Source: CAD feature listing. Evaluate the final solid. Frame: model axes, mm. Give positions to 0.01 mm unless a question says otherwise; leave off trailing zeros. Order: outer loops, then holes, each group sorted by start corner. A loop starts at its lowest first (then second) coordinate and runs counter-clockwise, first axis right, second up. Notation, with made-up numbers: M 28.5,18.25 L 80.5,18.25 A30 cw 80.5,40.25 Z; hole C 51.5,55 d5. An arc over 180 degrees is marked long. Return JSON: item names as keys, results as strings.
from build123d import *

# Parameters (mm, degrees)
SKETCH2_W           = 20
SKETCH2_H           = 20
BOSS_EXTRUDE1_DEPTH = 20
SKETCH3_R           = 2
CUT_EXTRUDE2_DEPTH  = 1.5
SKETCH4_R           = 2
CUT_EXTRUDE4_DEPTH  = 1.5
SKETCH5_R           = 2
CUT_EXTRUDE5_DEPTH  = 1.5
SKETCH6_R           = 2
CUT_EXTRUDE6_DEPTH  = 1.5
SKETCH7_R           = 2
CUT_EXTRUDE7_DEPTH  = 1.5
SKETCH8_R           = 2
CUT_EXTRUDE8_DEPTH  = 1.5
SKETCH9_R           = 2
CUT_EXTRUDE9_DEPTH  = 1.5


with BuildPart() as part:
    # Sketch2 → Boss-Extrude1 (new body)
    with BuildSketch(Plane.XY):
        with Locations((0, 10)):
            Rectangle(SKETCH2_W, SKETCH2_H)
    extrude(amount=BOSS_EXTRUDE1_DEPTH)

    # Sketch3 → Cut-Extrude2 (cut)
    with BuildSketch(Plane(origin=(0, 0, 0), x_dir=(-1, 0, 0), z_dir=(0, 0, -1))):
        with Locations((0, 11.387488096)):
            Circle(SKETCH3_R)
    extrude(amount=-CUT_EXTRUDE2_DEPTH, mode=Mode.SUBTRACT)

    # Sketch4 → Cut-Extrude4 (cut)
    with BuildSketch(Plane.XY.offset(20)):
        with Locations((-6.679680773, 3.199433654)):
            Circle(SKETCH4_R)
        with Locations((-6.679680773, 9.585684456)):
            Circle(SKETCH4_R)
        with Locations((-6.679680773, 15.895974219)):
            Circle(SKETCH4_R)
        with Locations(Location((5.94831499, 16.092405647, 0), (0, 0, 180))):
            Circle(SKETCH4_R)
        with Locations(Location((6.144583567, 9.785168888, 0), (0, 0, 180))):
            Circle(SKETCH4_R)
        with Locations(Location((6.343214755, 3.402007841, 0), (0, 0, 180))):
            Circle(SKETCH4_R)
    extrude(amount=-CUT_EXTRUDE4_DEPTH, mode=Mode.SUBTRACT)

    # Sketch5 → Cut-Extrude5 (cut)
    with BuildSketch(Plane.XZ):
        with Locations(Location((-7.031123571, 4.41764723, 0), (0, 0, 270))):
            Circle(SKETCH5_R)
        with Locations(Location((-7.031123571, 13.242962798, 0), (0, 0, 270))):
            Circle(SKETCH5_R)
        with Locations(Location((7.031123571, 13.242962798, 0), (0, 0, 90))):
            Circle(SKETCH5_R)
        with Locations(Location((7.031123571, 4.41764723, 0), (0, 0, 90))):
            Circle(SKETCH5_R)
    extrude(amount=-CUT_EXTRUDE5_DEPTH, mode=Mode.SUBTRACT)

    # Sketch6 → Cut-Extrude6 (cut)
    with BuildSketch(Plane(origin=(0, 20, 0), x_dir=(1, 0, 0), z_dir=(0, 1, 0))):
        with Locations(Location((-6.836211915, -14.945689643, 0), (0, 0, 270))):
            Circle(SKETCH6_R)
        with Locations(Location((3.056286481, -5.000631722, 0), (0, 0, 270))):
            Circle(SKETCH6_R)
    extrude(amount=-CUT_EXTRUDE6_DEPTH, mode=Mode.SUBTRACT)

    # Sketch7 → Cut-Extrude7 (cut)
    with BuildSketch(Plane.ZY.offset(10)):
        with Locations((15.664719218, 3.42791907)):
            Circle(SKETCH7_R)
        with Locations((6.506483369, 3.42791907)):
            Circle(SKETCH7_R)
        with Locations(Location((6.506483369, 15.851101107, 0), (0, 0, 180))):
            Circle(SKETCH7_R)
        with Locations(Location((15.664719218, 15.851101107, 0), (0, 0, 180))):
            Circle(SKETCH7_R)
    extrude(amount=-CUT_EXTRUDE7_DEPTH, mode=Mode.SUBTRACT)

    # Sketch8 → Cut-Extrude8 (cut)
    with BuildSketch(Plane.ZY.offset(10)):
        with Locations((10.73729624, 9.476774356)):
            Circle(SKETCH8_R)
    extrude(amount=-CUT_EXTRUDE8_DEPTH, mode=Mode.SUBTRACT)

    # Sketch9 → Cut-Extrude9 (cut)
    with BuildSketch(Plane(origin=(10, 0, 0), x_dir=(0, 0, -1), z_dir=(1, 0, 0))):
        with Locations((-16.749886235, 16.691371863)):
            Circle(SKETCH9_R)
        with Locations((-10.039394763, 9.986036972)):
            Circle(SKETCH9_R)
        with Locations((-4.265304833, 3.925944784)):
            Circle(SKETCH9_R)
    extrude(amount=-CUT_EXTRUDE9_DEPTH, mode=Mode.SUBTRACT)


solid = part.part
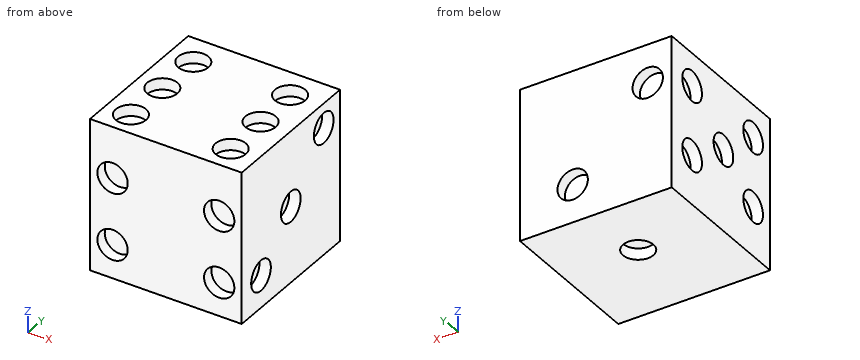
1. Ray query, probe 1 along Z at (x, y) = (5.75, 10.25); probe 2 along Y at (x, z) = (7, 14.25); probe 3 along X at (y, z) = (5.5, 3.5). Return the intervals inside material, ascending.
Evaluation:
{"probe 1": "z = 0 to 18.5", "probe 2": "y = 1.5 to 20", "probe 3": "x = -10 to 8.5"}
2. Section query A-A (x = 0). Return loops of the section in (y, z).
Evaluation:
{"outline": "M 0,0 L 9.39,0 L 9.39,1.5 L 13.39,1.5 L 13.39,0 L 20,0 L 20,20 L 0,20 Z"}
3. Section query B-B (y = 9). Return loops of the section in (x, z).
Evaluation:
{"outline": "M -10,0 L 10,0 L 10,8.3 L 8.5,8.3 L 8.5,11.78 L 10,11.78 L 10,20 L 7.98,20 L 7.98,18.5 L 4.31,18.5 L 4.31,20 L -4.77,20 L -4.77,18.5 L -8.59,18.5 L -8.59,20 L -10,20 L -10,12.68 L -8.5,12.68 L -8.5,8.79 L -10,8.79 Z"}
4. Section query C-C (z = 16). Return loops of the section in (x, y), then the cut area to 3 significant figures.
Evaluation:
{"outline": "M -10,0 L 10,0 L 10,14.84 L 8.5,14.84 L 8.5,18.55 L 10,18.55 L 10,20 L -5.14,20 L -5.14,18.5 L -8.54,18.5 L -8.54,20 L -10,20 L -10,17.82 L -8.5,17.82 L -8.5,13.88 L -10,13.88 L -10,5.4 L -8.5,5.4 L -8.5,1.46 L -10,1.46 Z", "area": "378 mm^2"}
5. First-contact query: pin 1 (1.2 mm diameter, centred on x = 7, z = 12.5, fed in from -Y); pin 2 (2.5 mm diameter, centred on y = 9.99, z = 10.04, fed in from +X); pin 3 (3 mm diameter, centred on x = -6.5, y = 10, fed in from +Z). Flat tips, straight axial feed; report the tip coordinate or a pass-through.
Evaluation:
{"pin 1": "stops at y = 1.5", "pin 2": "stops at x = 8.5", "pin 3": "stops at z = 18.5"}
